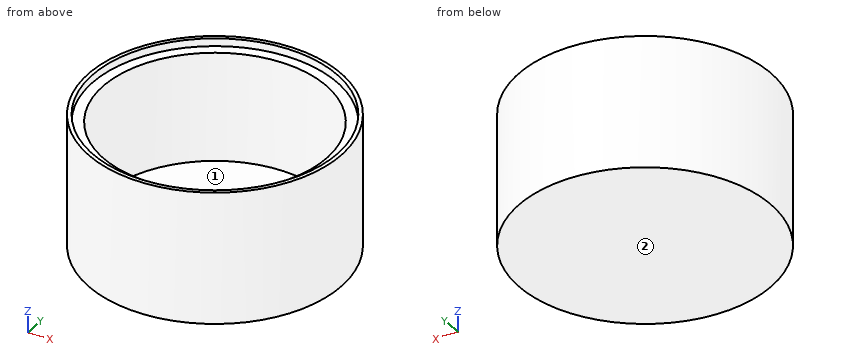
from build123d import *

# Parameters (mm, degrees)
F0_R     = 31.5
F0_R_2   = 28.75
F1_DEPTH = 28
F0_R_3   = 32.5
F2_DEPTH = 30
F3_DEPTH = 4


with BuildPart() as f1:
    # F0 (on Top) → F1 (new body)
    with BuildSketch(Plane.XY):
        Circle(F0_R)
        Circle(F0_R_2, mode=Mode.SUBTRACT)
    extrude(amount=F1_DEPTH)

    # F0 (on Top) → F2 (join)
    with BuildSketch(Plane.XY):
        Circle(F0_R_3)
        Circle(F0_R, mode=Mode.SUBTRACT)
    extrude(amount=F2_DEPTH)

    # F0 (on Top) → F3 (join)
    with BuildSketch(Plane.XY):
        Circle(F0_R_3)
        Circle(F0_R, mode=Mode.SUBTRACT)
        Circle(F0_R)
        Circle(F0_R_2, mode=Mode.SUBTRACT)
        Circle(F0_R_2)
    extrude(amount=-F3_DEPTH)


solid = f1.part
Verification items for the finished model (mm, model axes). Face numbers are marked on the shaded views. A direction names the side the tool comes from. Coordinates: 2 decimals unless noted, no trailing zeros. Write each loop counter-clockwise with the first axis right and the second up, starting at its lowest first coordinate (ties: lowest second). Pieces come first, ordered by that corner, then holes. Notation, with made-up numbers: (83, 81.5) -> (108, 81.5) arc R12 ccw to (108, 99.5) -> close; hole circle Ø5 at (58, 7.25). An arc over 180 degrees is marked (long way). One line per item, written item: value. Start each with the question number.
Q1. Cross-section at A-A on y = 0. Enter the section's corners in (x, z).
Q2. Thickness scan on L1, parallel to Y at x = 0, z = 29.45; L2, parallel to Z at x = 17.5, y = 0; L3, parallel to X at y = -4.5, z = 18.5. Record the ranges inside material, lowest first. Write a range as from..to.
Q3. Go/stop test with flat-tipped pins: P1, Ø3, axis at x = -17.5, y = -2.5, coming from the +Z side; P2, Ø2, axis at y = -9.5, z = 20, coming from the +X side; P3, Ø1.5, axis at x = -9.5, z = 23.5, coming from the +Y side. Record where each tip stops, or that it passes through.
Q4. Access from +Z, -Z, +X, -X, +Y, -Y to the whole of each face (thin tool, end or side, straight path). Record for the marked faces 1 and 2.
Checked values:
1. outline: (-32.5, -4) -> (32.5, -4) -> (32.5, 30) -> (31.5, 30) -> (31.5, 28) -> (28.75, 28) -> (28.75, 0) -> (-28.75, 0) -> (-28.75, 28) -> (-31.5, 28) -> (-31.5, 30) -> (-32.5, 30) -> close
2. L1: y = -32.5..-31.5, 31.5..32.5
2. L2: z = -4..0
2. L3: x = -32.19..-28.4, 28.4..32.19
3. P1: stops at z = 0
3. P2: stops at x = 31.37
3. P3: stops at y = 31.3
4. face 1: +Z
4. face 2: -Z, +X, -X, +Y, -Y
